from build123d import *

# Parameters (mm, degrees)
PAD_DEPTH         = 10
THICKNESS_T       = 1
SKETCH001_W       = 15
SKETCH001_H       = 10
SKETCH001_W_2     = 143
POCKET_DEPTH      = 5
POCKET_DEPTH_BACK = -5
SKETCH002_W       = 191
SKETCH002_H       = 10
POCKET001_DEPTH   = 17
FILLET_R          = 3


with BuildPart() as part:
    # Sketch → Pad (new body)
    with BuildSketch(Plane.XY):
        with BuildLine():
            Line((-76.5, 43.5), (76.5, 43.5))
            ThreePointArc((94.5, 25.5), (89.227922, 38.227922), (76.5, 43.5))
            Line((94.5, 25.5), (94.5, -25.5))
            ThreePointArc((76.5, -43.5), (89.227922, -38.227922), (94.5, -25.5))
            Line((76.5, -43.5), (-76.5, -43.5))
            ThreePointArc((-94.5, -25.5), (-89.227922, -38.227922), (-76.5, -43.5))
            Line((-94.5, -25.5), (-94.5, 25.5))
            ThreePointArc((-76.5, 43.5), (-89.227922, 38.227922), (-94.5, 25.5))
        make_face()
    extrude(amount=PAD_DEPTH)

    # Thickness
    thickness_openings = [part.faces().sort_by_distance(p)[0] for p in [
        (0, 0, 10),
    ]]
    offset(amount=THICKNESS_T, openings=thickness_openings)

    # Sketch001 (on Face5 of Thickness) → Pocket (cut, two sides)
    with BuildSketch(Plane(origin=(0, -43.5, 0), x_dir=(-1, 0, 0), z_dir=(0, 1, 0))) as pocket_sk:
        with Locations((79, 5)):
            Rectangle(SKETCH001_W, SKETCH001_H)
        with Locations((-79, 5)):
            Rectangle(SKETCH001_W, SKETCH001_H)
        with Locations((0, 5)):
            Rectangle(SKETCH001_W_2, SKETCH001_H)
    extrude(amount=-POCKET_DEPTH, mode=Mode.SUBTRACT)
    extrude(pocket_sk.sketch, amount=-POCKET_DEPTH_BACK, mode=Mode.SUBTRACT)

    # Sketch002 (on Face15 of Thickness) → Pocket001 (cut)
    with BuildSketch(Plane.XZ.offset(44.5)):
        with Locations((0, 5)):
            Rectangle(SKETCH002_W, SKETCH002_H)
    extrude(amount=-POCKET001_DEPTH, mode=Mode.SUBTRACT)

    # Fillet
    fillet_edges = [part.edges().sort_by_distance(p)[0] for p in [
        (-94.891494, -27.5, 10),
        (94.891494, -27.5, 10),
    ]]
    fillet(fillet_edges, radius=FILLET_R)


solid = part.part
Input: part model. Units: mm. Frame: model coordinates. A direction names the side the tool comes from. Coordinates: 2 decimals unless noted, no trailing zeros. Write each loop counter-clockwise with the first axis right and the second up, starting at its lowest first coordinate (ties: lowest second). Pieces come first, ordered by that corner, then holes. Notation, with made-up numbers: M 50.5,10.25 L 97.5,10.25 A24 cw 97.5,25.25 Z; hole C 33,58.5 d1. An arc over 180 degrees is marked long. Answer as a JSON object with one key per item and string values. Group by question number.
(1) Section C-C on y = 9.5. Output: boundary loops of the cut face in (x, z).
(2) Ray query, line 1 along X through (y, z) = (-10, 5.5); line 2 along Z through (x, y) = (-61, 5); line 3 along Y through (x, z) = (66.5, 8.5). Return the intervals inside material, ascending. Write a range as [from, to].
(3) Section A-A on x = -46.5. Output: boundary loops of the cut face in (y, z).
(4) Contact query for flat-ended pins moving along their axis: P1, Ø2, axis at x = 10.5, z = 5, coming from the -Y side; P2, Ø6, axis at x = -27.5, z = 0.5, coming from the -Y side; P3, Ø1, axis at x = -3.5, y = 10.5, coming from the +Z side. Output: stop coordinate, or through.
(5) Set-up query: faces 1 (the face through (1, 1, -1)), 2 (the face through (-1, 43.5, 5)). Return all of +Z, -Z, +X, -X, +Y, -Y with unobstructed straight access to the full face (end or side cutting, diameter ignored); none if empty.
(6) Section B-B on z = 3.5. Output: boundary loops of the cut face in (x, y).
Result set:
{
 "1": {"outline": "M -95.5,0 A1 ccw -94.5,-1 L 94.5,-1 A1 ccw 95.5,0 L 95.5,10 L 94.5,10 L 94.5,0 L -94.5,0 L -94.5,10 L -95.5,10 Z"},
 "2": {"line 1": "x = [-95.5, -94.5], [94.5, 95.5]", "line 2": "z = [-1, 0]", "line 3": "y = [43.5, 44.5]"},
 "3": {"outline": "M -44.5,0 A1 ccw -43.5,-1 L 43.5,-1 A1 ccw 44.5,0 L 44.5,10 L 43.5,10 L 43.5,0 Z"},
 "4": {"P1": "stops at y = 43.5", "P2": "stops at y = -44.5", "P3": "stops at z = 0"},
 "5": {"face 1": "-Z, +X, -X, +Y, -Y", "face 2": "+Z, -Y"},
 "6": {"outline": "M -95.5,-25.5 A19 ccw -95.39,-27.5 L -94.39,-27.5 A18 cw -94.5,-25.5 L -94.5,25.5 A18 cw -76.5,43.5 L 76.5,43.5 A18 cw 94.5,25.5 L 94.5,-25.5 A18 cw 94.39,-27.5 L 95.39,-27.5 A19 ccw 95.5,-25.5 L 95.5,25.5 A19 ccw 76.5,44.5 L -76.5,44.5 A19 ccw -95.5,25.5 Z"}
}
